Can you work these out from the model? Positions are in its coordinate system, mm. A direction names the side the tool comes from. Coordinates: 2 decimals unless noted, no trailing zeros. Loops run counter-clockwise (first coordinate to the right, second up) from the corner with the lowest first, then second, coordinate; pieces in that order, holes last.
```python
from build123d import *

# Parameters (mm, degrees)
BOSS_EXTRUDE1_DEPTH      = 7.5
BOSS_EXTRUDE1_DEPTH_BACK = 7.5
FILLET1_R                = 5


with BuildPart() as part:
    # Sketch1 → Boss-Extrude1 (new, two sides: drawn at the far end of the back side and taken through both)
    with BuildSketch(Plane.XY.offset(-BOSS_EXTRUDE1_DEPTH_BACK)):
        Polygon((-20, 20), (20, 20), (20, 0), (10, 0), (10, 2.5), (17.5, 10), (17.5, 17.5), (-17.5, 17.5), (-17.5, 10), (-10, 2.5), (-10, 0), (-20, 0), align=None)
    extrude(amount=BOSS_EXTRUDE1_DEPTH + BOSS_EXTRUDE1_DEPTH_BACK)

    # Fillet1
    fillet1_edges = [part.edges().sort_by_distance(p)[0] for p in [
        (-20, 20, 0),
        (20, 20, 0),
        (10, 2.5, 0),
        (17.5, 10, 0),
        (17.5, 17.5, 0),
        (-17.5, 17.5, 0),
        (-17.5, 10, 0),
        (-10, 2.5, 0),
    ]]
    fillet(fillet1_edges, radius=FILLET1_R)


solid = part.part
```
(1) I want a section at B-B on y = 9.75. Write out the boundary of the cut face in (x, z).
Check values:
outline: (-20, -7.5) - (-16.93, -7.5) - (-16.93, 7.5) - (-20, 7.5) - close; (16.93, -7.5) - (20, -7.5) - (20, 7.5) - (16.93, 7.5) - close
(2) I'm going to push a flat-ended pin straight in: pin 1 (1 mm diameter, centred on x = 4, z = 2.5, fed in from -Y). Where does the tip first touch, or does it pass through?
Check values:
pin 1: stops at y = 17.5
(3) I want a section at D-D on x = -1. Write out the boundary of the cut face in (y, z).
Check values:
outline: (17.5, -7.5) - (20, -7.5) - (20, 7.5) - (17.5, 7.5) - close
(4) If I drill on probe 1 along X at (y, z) = (12.75, -4); probe 2 along Y at (x, z) = (-3.5, 3.5); probe 3 along X at (y, z) = (11.25, -2.75), over which ranges is the centre line in solid material (lowest first)?
Check values:
probe 1: x = -20 to -17.49, 17.49 to 20
probe 2: y = 17.5 to 20
probe 3: x = -20 to -17.43, 17.43 to 20
(5) I want a section at A-A on x = 12. Write out the boundary of the cut face in (y, z).
Check values:
outline: (0, -7.5) - (4.5, -7.5) - (4.5, 7.5) - (0, 7.5) - close; (17.5, -7.5) - (20, -7.5) - (20, 7.5) - (17.5, 7.5) - close
(6) I want a section at C-C on z = -1. Write out the boundary of the cut face in (x, y).
Check values:
outline: (-20, 0) - (-10, 0) - (-10, 0.43) arc R5 ccw to (-11.46, 3.96) - (-16.04, 8.54) arc R5 cw to (-17.5, 12.07) - (-17.5, 12.5) arc R5 cw to (-12.5, 17.5) - (12.5, 17.5) arc R5 cw to (17.5, 12.5) - (17.5, 12.07) arc R5 cw to (16.04, 8.54) - (11.46, 3.96) arc R5 ccw to (10, 0.43) - (10, 0) - (20, 0) - (20, 15) arc R5 ccw to (15, 20) - (-15, 20) arc R5 ccw to (-20, 15) - close
(7) If we mould it in two halves opening along X, with no side actions, what happens to faces 3 (the cylindrical face through (-18, 19, 0)), 4 (the flat face through (13.7, 6.2, -0.1)), 5 (the flat face through (20, 8, 0))? For each: released by +X, released by -X, zero draft, split by the parting line, or undercut.
Check values:
face 3: released by -X
face 4: undercut
face 5: released by +X
(8) Which directions (+Z, -Z, +X, -X, +Y, -Y) give clear straight access to the entire face, cutting with the end or side of a thin tool? Please do faces 1 (the cylindrical face through (16.07, 16, 0.11)), 2 (the flat face through (0, 20, 0)).
Check values:
face 1: +Z, -Z
face 2: +Z, -Z, +X, -X, +Y
